For this review, use the dimensioned drawing (mm, ordinates from the lowest corner) and the shaded views. Round coordinates to 2 decimals unless told otherwise and drop trailing zeros. Loops run counter-clockwise (first coordinate to the right, second up) from the corner with the lowest first, then second, coordinate; pieces in that order, holes last. Notation, with made-up numbers: (-2.5, -6) - (21.5, -6) arc R15 cw to (21.5, 10) - close; hole circle Ø1 at (41, 85). An arc over 180 degrees is marked (long way). Use one line per item in the form item = value. Start each with the question number.
(1) We need section C-C, the plane y = 45.5. Write out the cut boundary in (x, z).
(2) We need section A-A, the plane z = 250. Write out the cut boundary in (x, y), then the cut area to 3 significant figures.
(3) We need section B-B, the plane x = 371. Write out the cut boundary in (y, z), then the cut area to 3 significant figures.
(4) For pin 1 (23.5 mm diameter, centred on x = 50, z = 150, fed in from -Y), flat-tipped, find the tip position at first contact; note if it passes through.
(5) Wall thickness on probe 1 along X at (y, z) = (28, 250); probe 2 along X at (y, z) = (22, 150); probe 3 along Z at (x, y) = (368, 40): over which ranges is each line inside the solid? List them lowest first. Write a range as [from, to].
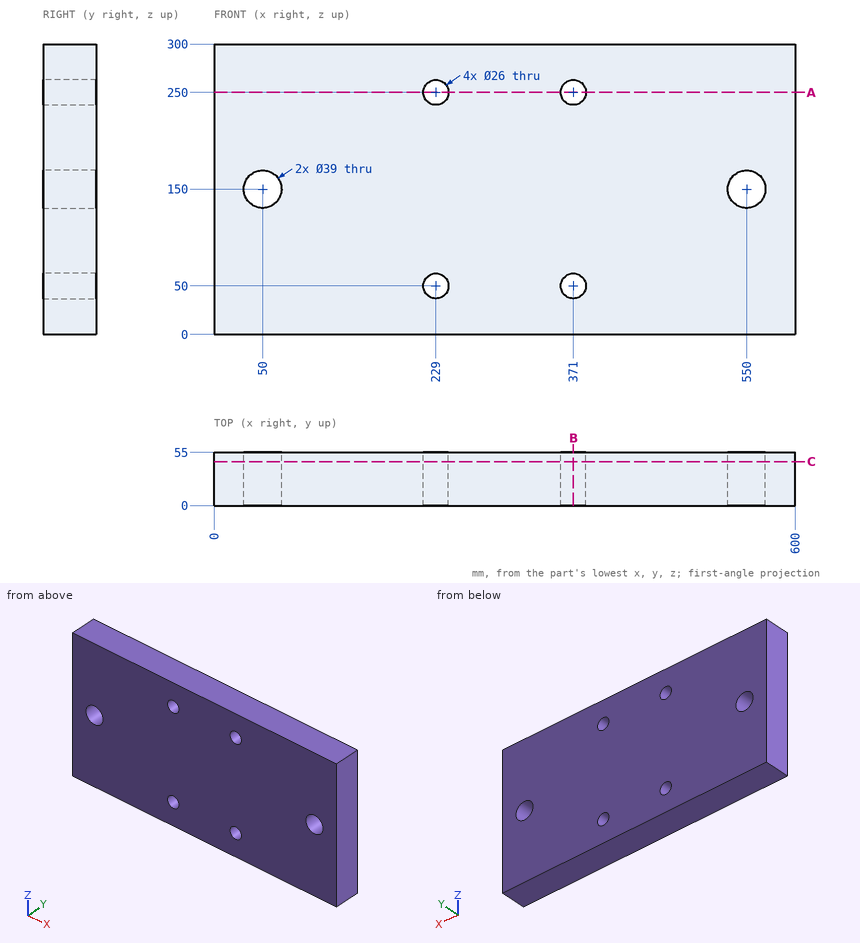
Data:
q1.outline = (0, 0) - (600, 0) - (600, 300) - (0, 300) - close; hole circle Ø39 at (50, 150); hole circle Ø26 at (229, 50); hole circle Ø26 at (229, 250); hole circle Ø26 at (371, 50); hole circle Ø26 at (371, 250); hole circle Ø39 at (550, 150)
q2.outline = (0, 0) - (216, 0) - (216, 55) - (0, 55) - close; (242, 0) - (358, 0) - (358, 55) - (242, 55) - close; (384, 0) - (600, 0) - (600, 55) - (384, 55) - close
q2.area = 30,100 mm^2
q3.outline = (0, 0) - (55, 0) - (55, 37) - (0, 37) - close; (0, 63) - (55, 63) - (55, 237) - (0, 237) - close; (0, 263) - (55, 263) - (55, 300) - (0, 300) - close
q3.area = 13,600 mm^2
q4.pin_1 = through
q5.probe_1 = [0, 216], [242, 358], [384, 600]
q5.probe_2 = [0, 30.5], [69.5, 530.5], [569.5, 600]
q5.probe_3 = [0, 37.35], [62.65, 237.35], [262.65, 300]
